Study the drawing (mm; zero at the part's minimum x, y, z) and answer. Coordinates: 2 decimals unless noted, no trailing zeros. Order: outer loops, then holes, each group sorted by start corner. A loop starts at its lowest first (then second) coordinate and runs counter-clockwise, first axis right, second up. Notation, with made-up numbers: M 89,47.25 L 145,47.25 A24 cw 145,73.25 Z; hole C 42.25,67.5 d2. An arc over 180 degrees is marked long. Put each result on its own line as item: value.
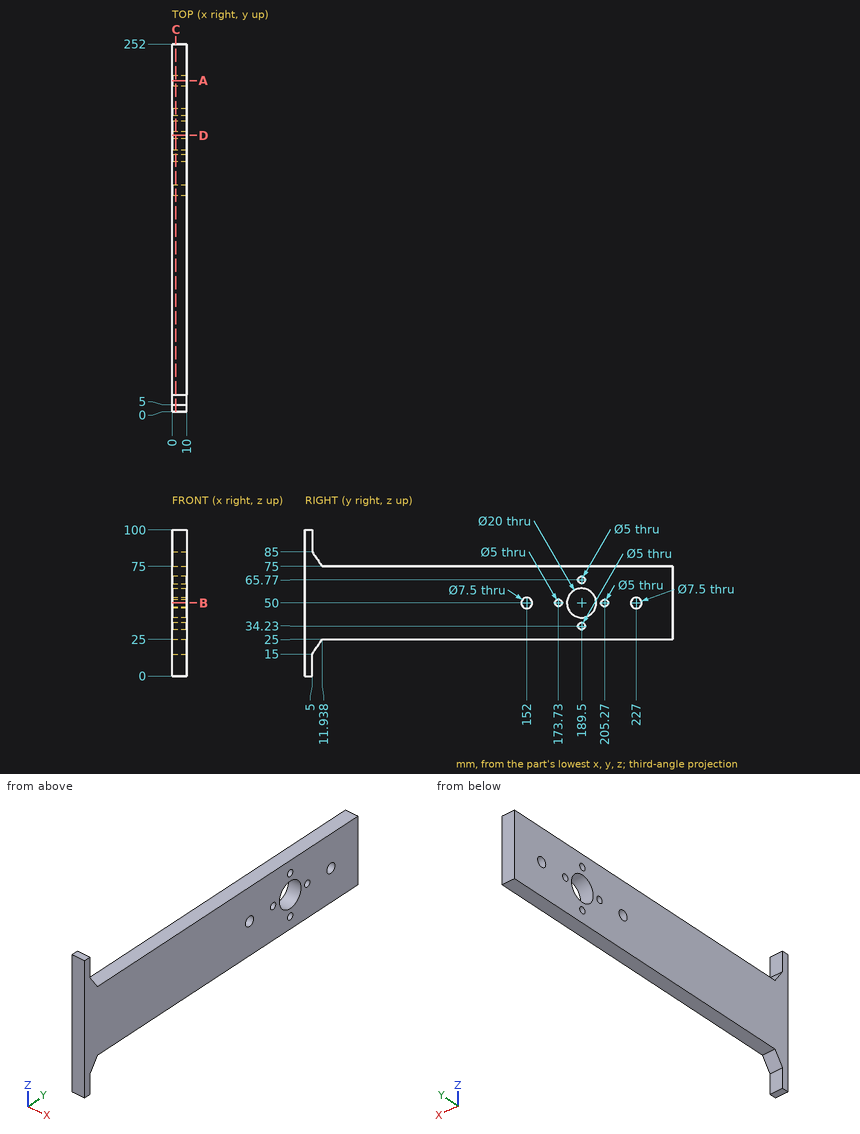
Q1. Given pin 1 (3 mm diameter, centred on x = 7.5, y = 60.5, fed in from +Z); pin 2 (5 mm diameter, centred on x = 5.5, y = 178, fed in from -Z); pin 3 (3 mm diameter, centred on y = 173.73, z = 50, fed in from +X), each flat-ended and moving along its own axis, determine where each tip first touches the part or whether it passes through.
Answers below:
pin 1: stops at z = 75
pin 2: stops at z = 25
pin 3: passes through
Q2. Find section A-A on y = 227. Write down the section's boundary in (x, z), plus the area to 3 significant figures.
Answers below:
outline: M 0,25 L 10,25 L 10,46.25 L 0,46.25 Z; M 0,53.75 L 10,53.75 L 10,75 L 0,75 Z
area: 425 mm^2
Q3. Find section C-C on x = 2.5. Write down the section's boundary in (y, z), plus the area to 3 significant figures.
Answers below:
outline: M 0,0 L 5,0 L 5,15 L 11.94,25 L 252,25 L 252,75 L 11.94,75 L 5,85 L 5,100 L 0,100 Z; hole C 152,50 d7.5; hole C 173.73,50 d5; hole C 189.5,50 d20; hole C 189.5,34.23 d5; hole C 189.5,65.77 d5; hole C 205.27,50 d5; hole C 227,50 d7.5
area: 12,400 mm^2
Q4. Consider line 1 along Y through (x, z) = (2.5, 50); line 2 along Z through (x, y) = (3.25, 205.27); line 3 along Z through (x, y) = (6, 227). Determine where each line is inside the solid, lowest interval first.
Answers below:
line 1: y = 0 to 148.25, 155.75 to 171.23, 176.23 to 179.5, 199.5 to 202.77, 207.77 to 223.25, 230.75 to 252
line 2: z = 25 to 47.5, 52.5 to 75
line 3: z = 25 to 46.25, 53.75 to 75
Q5. Find section B-B on z = 50. Write down the section's boundary in (x, y).
Answers below:
outline: M 0,0 L 10,0 L 10,148.25 L 0,148.25 Z; M 0,155.75 L 10,155.75 L 10,171.23 L 0,171.23 Z; M 0,176.23 L 10,176.23 L 10,179.5 L 0,179.5 Z; M 0,199.5 L 10,199.5 L 10,202.77 L 0,202.77 Z; M 0,207.77 L 10,207.77 L 10,223.25 L 0,223.25 Z; M 0,230.75 L 10,230.75 L 10,252 L 0,252 Z
Q6. Find section D-D on y = 189.5. Write down the section's boundary in (x, z).
Answers below:
outline: M 0,25 L 10,25 L 10,31.73 L 0,31.73 Z; M 0,36.73 L 10,36.73 L 10,40 L 0,40 Z; M 0,60 L 10,60 L 10,63.27 L 0,63.27 Z; M 0,68.27 L 10,68.27 L 10,75 L 0,75 Z
